from build123d import *

# Parameters (mm, degrees)
BOSS_EXTRUDE1_DEPTH        = 18
SKETCH2_R                  = 3
CUT_EXTRUDE1_DEPTH         = 38
F_12_0MM_DOWEL_HOLE1_D     = 12
F_12_0MM_DOWEL_HOLE1_DEPTH = 20
F_12_0MM_DOWEL_HOLE1_TIP   = 3.605163714


with BuildPart() as part:
    # Sketch1 → Boss-Extrude1 (new body)
    with BuildSketch(Plane(origin=(0, 0, 0), x_dir=(1, 0, 0), z_dir=(0, 1, 0))):
        Polygon((0, 60), (0, 0), (3.5, 0), (3.5, 2.5), (6, 2.5), (6, 5), (8.5, 5), (8.5, 7.5), (11, 7.5), (11, 10), (13.5, 10), (13.5, 12.5), (16, 12.5), (16, 15), (22, 15), (22, 12.5), (24.5, 12.5), (24.5, 10), (27, 10), (27, 7.5), (29.5, 7.5), (29.5, 5), (32, 5), (32, 2.5), (34.5, 2.5), (34.5, 0), (38, 0), (38, 60), align=None)
    extrude(amount=BOSS_EXTRUDE1_DEPTH)

    # Sketch2 → Cut-Extrude1 (cut)
    with BuildSketch(Plane(origin=(38, 0, 0), x_dir=(0, 0, -1), z_dir=(1, 0, 0))):
        with Locations((53, 9)):
            Circle(SKETCH2_R)
    extrude(amount=-CUT_EXTRUDE1_DEPTH, mode=Mode.SUBTRACT)

    # Ø12.0mm Dowel Hole1
    with Locations(Plane(origin=(19, 9, -60), x_dir=(-1, 0, 0), z_dir=(0, 0, -1))):
        with Locations((0, 0)):
            Hole(F_12_0MM_DOWEL_HOLE1_D / 2, depth=F_12_0MM_DOWEL_HOLE1_DEPTH)
            with Locations((0, 0, -(F_12_0MM_DOWEL_HOLE1_DEPTH + F_12_0MM_DOWEL_HOLE1_TIP / 2))):  # 118° drill point
                Cone(0, F_12_0MM_DOWEL_HOLE1_D / 2, F_12_0MM_DOWEL_HOLE1_TIP, mode=Mode.SUBTRACT)


solid = part.part
Input: part model. Units: mm. Frame: model coordinates. A direction names the side the tool comes from. Give positions to 0.01 mm unless a question says otherwise; leave off trailing zeros. Write each loop counter-clockwise with the first axis right and the second up, starting at its lowest first coordinate (ties: lowest second). Pieces come first, ordered by that corner, then holes. Notation, with made-up numbers: M 69.25,3 L 100.25,3 A8 ccw 100.25,7 Z; hole C 79.5,17 d11. An arc over 180 degrees is marked long. Write item = value, one per line. Start each with the question number.
1) Material intervals for line 1 along Y through (x, z) = (35.25, -53); line 2 along X through (y, z) = (9, -44.5); line 3 along Z through (x, y) = (9, 9), sorted ascending. Write a range as [from, to].
2) Draft query along Z for faces 4 (the conical face through (18.01, 9.31, -37.02)), 5 (the flat face through (19, 9, -15)), 6 (the cylindrical face through (31, 9, -50)), 7 (the flat face through (6, 9, -4)). Return one class per face: +Z half, -Z half, draft (parallel to the pull), parting line (faces both ways), or undercut.
3) Cut plane A-A on z = -53. Return the cut outline in (x, y), then the cut area to 3 significant figures.
4) First-contact query: pin 1 Ø3 at (x, y) = (24.5, 15) entering from +Z; pin 2 Ø5 at (y, z) = (7, -51.5) entering from -X; pin 3 Ø1 at (x, y) = (20.5, 7) entering from -Z; pin 4 Ø1.2 at (x, y) = (4.5, 7) entering from +Z. Flat tips, straight axial feed; report the tip coordinate or a pass-through.
5) Cut plane B-B on z = -45. Return the cut outline in (x, y), then the cut area to 3 significant figures.
6) Reachability of faces 1 (the cylindrical face through (7, 9, -50)), 2 (the flat face through (10, 9, -7.5)), 3 (the cylindrical face through (13.006, 9.264, -49.86)) from +Z, -Z, +X, -X, +Y, -Y: full face, straight path, thin tool, end or side. Return the list, or none.
7) Cut plane C-C on y = 7. Count the separate pieces of the cut face and the enclosed holes in it, then the cut area to 3 significant figures.
Solved:
q1.line_1 = [0, 6], [12, 18]
q1.line_2 = [0, 13], [25, 38]
q1.line_3 = [-60, -56], [-50, -7.5]
q2.face_4 = -Z half
q2.face_5 = +Z half
q2.face_6 = undercut
q2.face_7 = draft
q3.outline = M 0,0 L 38,0 L 38,6 L 24.2,6 A6 cw 13.8,6 L 0,6 Z; M 0,12 L 13.8,12 A6 cw 24.2,12 L 38,12 L 38,18 L 0,18 Z
q3.area = 412 mm2
q4.pin_1 = -10
q4.pin_2 = 0
q4.pin_3 = -38.2
q4.pin_4 = -2.5
q5.outline = M 0,0 L 38,0 L 38,18 L 0,18 Z; hole C 19,9 d12
q5.area = 571 mm2
q6.face_1 = +X, -X
q6.face_2 = +Z, +Y, -Y
q6.face_3 = -Z
q7.separate_pieces = 3
q7.enclosed_holes = 0
q7.area = 1,640 mm2
